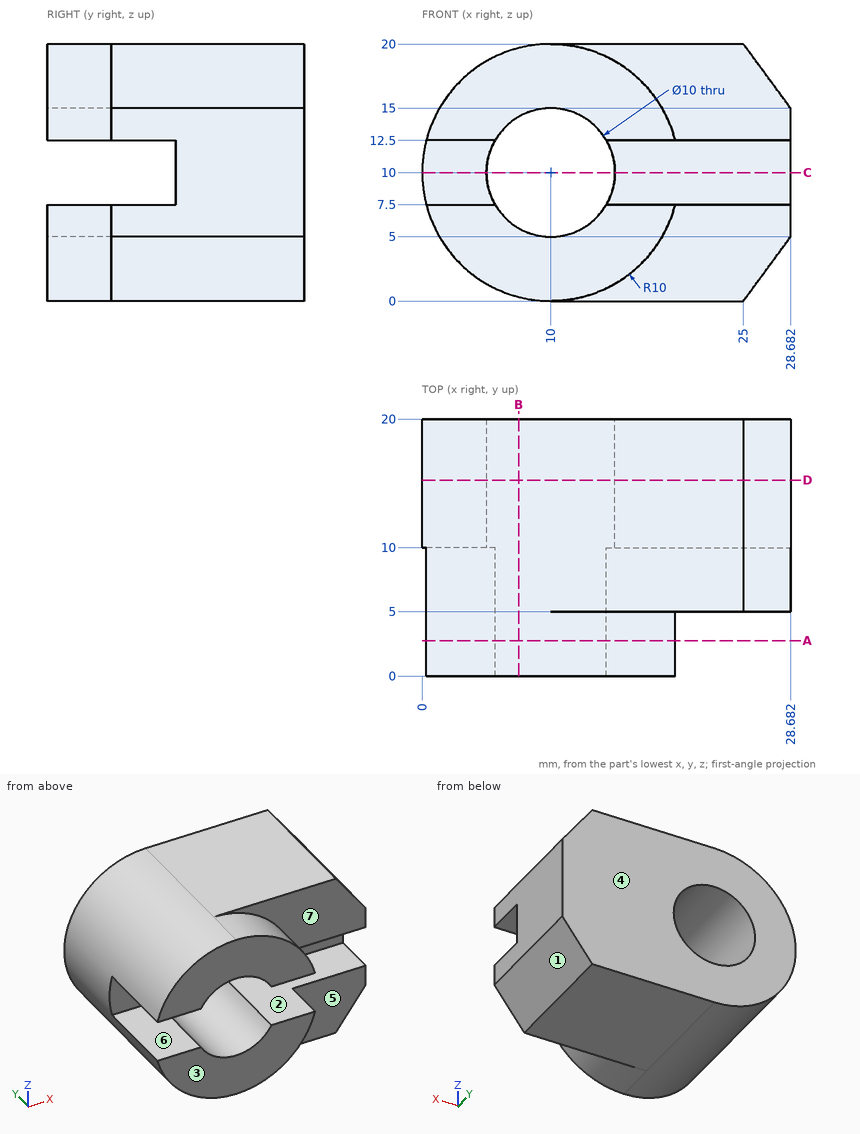
Geometry check sheet. Reference: drawing and pictorial views, mm from the part's lowest x, y, z. A direction names the side the tool comes from. Round coordinates to 2 decimals unless told otherwise and drop trailing zeros. Write each loop counter-clockwise with the first axis right and the second up, starting at its lowest first coordinate (ties: lowest second). Pieces come first, ordered by that corner, then holes.
Item 1: Section check C-C (z = 10). Record the boundary of the cut face in (x, y), plus the area to 3 significant figures.
Determined:
outline: (0, 10) - (5, 10) - (5, 20) - (0, 20) - close; (15, 10) - (28.68, 10) - (28.68, 20) - (15, 20) - close
area: 187 mm2
Item 2: Material ranges on line 1 along Z through (x, y) = (10, 15.5); line 2 along Y through (x, z) = (24.75, 8.5); line 3 along Y through (x, z) = (26.5, 3), recorded low to high.
Determined:
line 1: z = 0 to 5, 15 to 20
line 2: y = 10 to 20
line 3: y = 5 to 20
Item 3: Access from +Z, -Z, +X, -X, +Y, -Y to the whole of each face (thin tool, end or side, straight path). Record for the marked faces 4, 5, 6 and 7.
Determined:
face 4: +Z, -Z, +X, -X, +Y
face 5: -Z, +X, -Y
face 6: +X, -X, -Y
face 7: +Z, +X, -Y
Item 4: Mould release check, pull along Z, two halves, no side actions. Record for the marked faces 1, 2 and 3: +Z half, -Z half, draft (parallel to the pull), parting line (faces both ways), or undercut.
Determined:
face 1: -Z half
face 2: undercut
face 3: draft
Item 5: Go/stop test with flat-tipped pins: pin 1 Ø1.6 at (x, y) = (4, 6.5) entering from +Z; pin 2 Ø8 at (x, z) = (10, 10) entering from -Y; pin 3 Ø1.5 at (x, z) = (25, 9) entering from -Y; pin 4 Ø4.5 at (x, y) = (2, 6) entering from -Z. Record where each tip stops, or that it passes through.
Determined:
pin 1: stops at z = 18.54
pin 2: passes through
pin 3: stops at y = 10
pin 4: stops at z = 1.82
Item 6: Section check B-B (x = 7.5). Record the boundary of the cut face in (y, z).
Determined:
outline: (0, 0.32) - (20, 0.32) - (20, 5.67) - (0, 5.67) - close; (0, 14.33) - (20, 14.33) - (20, 19.68) - (0, 19.68) - close
Item 7: Section check A-A (y = 2.75). Record the boundary of the cut face in (x, z).
Determined:
outline: (0.32, 7.5) arc R10 ccw to (19.68, 7.5) - (14.33, 7.5) arc R5 cw to (5.67, 7.5) - close; (0.32, 12.5) - (5.67, 12.5) arc R5 cw to (14.33, 12.5) - (19.68, 12.5) arc R10 ccw to start
Item 8: Section check D-D (y = 15.25). Record the boundary of the cut face in (x, z).
Determined:
outline: (10, 0) - (25, 0) - (28.68, 5) - (28.68, 15) - (25, 20) - (10, 20) arc R10 ccw to start; hole circle Ø10 at (10, 10)
